from build123d import *

# Parameters (mm, degrees)
F0_R     = 76.139755
F1_DEPTH = 151.638
F2_R     = 67.495024
F3_DEPTH = 149.098
F4_R     = 68.23758
F4_R_2   = 59.894351
F5_DEPTH = 25.4
F6_R     = 60.764982
F7_DEPTH = 145.542


with BuildPart() as f1:
    # F0 (on Top) → F1 (new body)
    with BuildSketch(Plane.XY):
        Circle(F0_R)
    extrude(amount=F1_DEPTH)

    # F2 (on Top) → F3 (join)
    with BuildSketch(Plane.XY):
        Circle(F2_R)
    extrude(amount=F3_DEPTH)

    # F4 (on Top) → F5 (cut)
    with BuildSketch(Plane.XY):
        Circle(F4_R)
        Circle(F4_R_2, mode=Mode.SUBTRACT)
    extrude(amount=-F5_DEPTH, mode=Mode.SUBTRACT)

    # F6 (on Top) → F7 (cut)
    with BuildSketch(Plane.XY):
        Circle(F6_R)
    extrude(amount=F7_DEPTH, mode=Mode.SUBTRACT)


solid = f1.part
Geometry: final body of the model. Coordinates: model frame, mm. A direction names the side the tool comes from. Coordinates: 2 decimals unless noted, no trailing zeros. Loops run counter-clockwise (first coordinate to the right, second up) from the corner with the lowest first, then second, coordinate; pieces in that order, holes last. Notation, with made-up numbers: M 61,62.5 L 109,62.5 A30 ccw 109,93.5 Z; hole C 25,40.5 d3. An arc over 180 degrees is marked long. One line per item, written item: value. Start each with the question number.
1) Cut plane C-C (z = 116.5). Return loops of the section in (x, y), then the cut area to 3 significant figures.
2) Material intervals for L1, parallel to Y at x = 0, z = 68; L2, parallel to Z at x = -33, y = 48; L3, parallel to X at y = -2, z = 99.5, sorted ascending. Write a range as from..to.
3) Draft query along Y for faces 3 (the cylindrical face through (-16.51, -74.33, 74.76)), 4 (the flat face through (-51.1, -33.5, 0)), 5 (the cylindrical face through (32.667, 51.237, 71.752)). Return one class per face: released by +Y, released by -Y, zero draft, split by the parting line, or undercut.
4) Cut plane A-A (x = 0). Return loops of the section in (y, z), then the cut area to 3 significant figures.
5) Cut plane D-D (x = -64). Return loops of the section in (y, z), then the cut area to 3 significant figures.
6) Reachability of faces 1 (the flat face through (-1, 1, 151.638)), 2 (the flat face through (-1, 1, 145.542)) from +Z, -Z, +X, -X, +Y, -Y: full face, straight path, thin tool, end or side. Return the list, or none.
7) Pin query (flat end, axial travel): P1, Ø2, axis at y = -11, z = 77, coming from the +X side; P2, Ø8, axis at y = 22.5, z = 90.5, coming from the +X side; P3, Ø1, axis at x = -49, z = 112, coming from the +Y side. Return the tip coordinate at first contact, or that it passes through.
Evaluation:
1. outline: C 0,0 d152.28; hole C 0,0 d121.53
1. area: 6,610 mm^2
2. L1: -76.14..-60.76, 60.76..76.14
2. L2: 145.54..151.64
2. L3: -76.11..-60.73, 60.73..76.11
3. face 3: split by the parting line
3. face 4: zero draft
3. face 5: undercut
4. outline: M -76.14,0 L -60.76,0 L -60.76,145.54 L 60.76,145.54 L 60.76,0 L 76.14,0 L 76.14,151.64 L -76.14,151.64 Z
4. area: 5,400 mm^2
5. outline: M -41.25,0 L 41.25,0 L 41.25,151.64 L -41.25,151.64 Z
5. area: 12,500 mm^2
6. face 1: +Z, +X, -X, +Y, -Y
6. face 2: -Z
7. P1: x = 75.48
7. P2: x = 73.86
7. P3: y = 58.69
